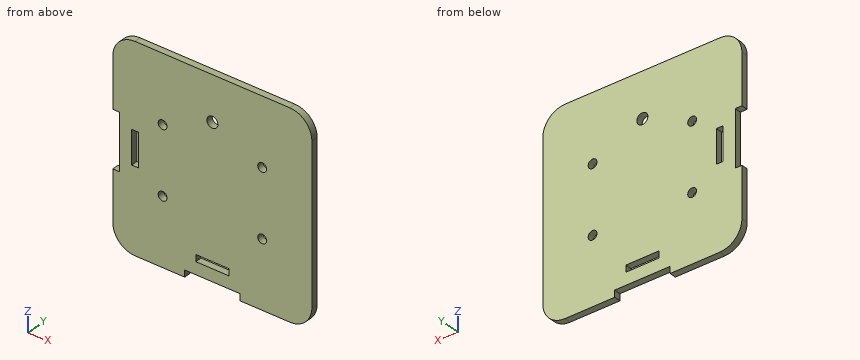
from build123d import *

# Parameters (mm, degrees)
BOSS_EXTRUDE1_DEPTH = 3
SKETCH2_R           = 2
CUT_EXTRUDE1_DEPTH  = 3
SKETCH3_W           = 15
SKETCH3_H           = 3
SKETCH3_W_2         = 3
SKETCH3_H_2         = 15
CUT_EXTRUDE2_DEPTH  = 10
SKETCH4_R           = 2.5
CUT_EXTRUDE3_DEPTH  = 14


with BuildPart() as part:
    # Sketch1 → Boss-Extrude1 (new body)
    with BuildSketch(Plane(origin=(0, 0, 0), x_dir=(1, 0, 0), z_dir=(0, 1, 0))):
        with BuildLine():
            Line((-35, -45), (35, -45))
            ThreePointArc((35, -45), (42.071067812, -42.071067812), (45, -35))
            Line((45, -35), (45, 35))
            ThreePointArc((45, 35), (42.071067812, 42.071067812), (35, 45))
            Line((35, 45), (12.5, 45))
            Line((12.5, 45), (12.5, 42))
            Line((12.5, 42), (-12.5, 42))
            Line((-12.5, 42), (-12.5, 45))
            Line((-12.5, 45), (-35, 45))
            ThreePointArc((-35, 45), (-42.071067812, 42.071067812), (-45, 35))
            Line((-45, 35), (-45, 12.5))
            Line((-45, 12.5), (-42, 12.5))
            Line((-42, 12.5), (-42, -12.5))
            Line((-42, -12.5), (-45, -12.5))
            Line((-45, -12.5), (-45, -35))
            ThreePointArc((-45, -35), (-42.071067812, -42.071067812), (-35, -45))
        make_face()
    extrude(amount=BOSS_EXTRUDE1_DEPTH)

    # Sketch2 → Cut-Extrude1 (cut)
    with BuildSketch(Plane(origin=(0, 3, 0), x_dir=(1, 0, 0), z_dir=(0, 1, 0))):
        with Locations(Location((-22.5, 15, 0), (0, 0, 270))):
            Circle(SKETCH2_R)
        with Locations(Location((22.5, 15, 0), (0, 0, 90))):
            Circle(SKETCH2_R)
        with Locations(Location((22.5, -15, 0), (0, 0, 270))):
            Circle(SKETCH2_R)
        with Locations(Location((-22.5, -15, 0), (0, 0, 90))):
            Circle(SKETCH2_R)
    extrude(amount=-CUT_EXTRUDE1_DEPTH, mode=Mode.SUBTRACT)

    # Sketch3 → Cut-Extrude2 (cut)
    with BuildSketch(Plane(origin=(0, 3, 0), x_dir=(1, 0, 0), z_dir=(0, 1, 0))):
        with Locations((0, 35)):
            Rectangle(SKETCH3_W, SKETCH3_H)
        with Locations((-35, 0)):
            Rectangle(SKETCH3_W_2, SKETCH3_H_2)
    extrude(amount=-CUT_EXTRUDE2_DEPTH, mode=Mode.SUBTRACT)

    # Sketch4 → Cut-Extrude3 (cut)
    with BuildSketch(Plane(origin=(0, 3, 0), x_dir=(1, 0, 0), z_dir=(0, 1, 0))):
        with Locations(Location((0, -25, 0), (0, 0, 270))):
            Circle(SKETCH4_R)
    extrude(amount=-CUT_EXTRUDE3_DEPTH, mode=Mode.SUBTRACT)


solid = part.part
Build history of the part. All positions in model axes, mm. Give positions to 0.01 mm unless a question says otherwise; leave off trailing zeros. Write each loop counter-clockwise with the first axis right and the second up, starting at its lowest first coordinate (ties: lowest second). Pieces come first, ordered by that corner, then holes. Notation, with made-up numbers: (-10, 52) - (46, 52) arc R18 cw to (46, 79) - close; hole circle Ø1 at (30, 45.25). An arc over 180 degrees is marked (long way). Use one line per item in the form item = value. Start each with the question number.
1. Drop flat-ended pins along their axis: pin 1 Ø1.5 at (x, y) = (-43.5, 1.5) entering from +Z; pin 2 Ø1.5 at (x, y) = (-43, 1.5) entering from -Z; pin 3 Ø1.5 at (y, z) = (1.5, 0) entering from -X. Give the stop position or say it passes through.
2. Band-saw the part on C-C on z = 25. Write the cut outline in (x, y), plus the area to 3 significant figures.
3. Band-saw the part on B-B on z = 15. Write the cut outline in (x, y), plus the area to 3 significant figures.
4. Probe line 1 (X direction, y = 2, z = -15); line 2 (Z direction, x = 4.5, y = 1.1). List the from-to ranges inside material, lowest first. Write a range as [from, to].
5. Band-saw the part on A-A on x = 22.5. Write the cut outline in (y, z), plus the area to 3 significant figures.
Conclusion:
q1.pin_1 = 41.32
q1.pin_2 = -41.89
q1.pin_3 = -42
q2.outline = (-45, 0) - (-2.5, 0) - (-2.5, 3) - (-45, 3) - close; (2.5, 0) - (45, 0) - (45, 3) - (2.5, 3) - close
q2.area = 255 mm²
q3.outline = (-45, 0) - (-24.5, 0) - (-24.5, 3) - (-45, 3) - close; (-20.5, 0) - (20.5, 0) - (20.5, 3) - (-20.5, 3) - close; (24.5, 0) - (45, 0) - (45, 3) - (24.5, 3) - close
q3.area = 246 mm²
q4.line_1 = [-45, -24.5], [-20.5, 20.5], [24.5, 45]
q4.line_2 = [-42, -36.5], [-33.5, 45]
q5.outline = (0, -45) - (3, -45) - (3, -17) - (0, -17) - close; (0, -13) - (3, -13) - (3, 13) - (0, 13) - close; (0, 17) - (3, 17) - (3, 45) - (0, 45) - close
q5.area = 246 mm²
